```python
from build123d import *

# Parameters (mm, degrees)
ENL_V_MAT_EXTRU_1_DEPTH = 8.5
ESQUISSE3_R             = 1.25
ENL_V_MAT_EXTRU_2_DEPTH = 4
CHANFREIN1_SIZE         = 0.5


with BuildPart() as part:
    # Esquisse1 → Révolution1 (revolve)
    with BuildSketch(Plane.XY, mode=Mode.PRIVATE) as r_volution1_sk:
        Polygon((4.25, 1), (13.5, 1), (13.5, 22), (13.6, 22), (13.6, 37), (4.5, 37), (4.5, 41.5), (2, 41.5), (2, 52.5), (0, 52.5), (0, 0), (4.25, 0), align=None)
    revolve(r_volution1_sk.sketch.rotate(Axis((0, 52.5, 0), (0, -1, 0)), 180), axis=Axis((0, 52.5, 0), (0, -1, 0)))

    # Esquisse2 → Enlèv. mat.-Extru.1 (cut)
    with BuildSketch(Plane(origin=(0, 52.5, 0), x_dir=(1, 0, 0), z_dir=(0, 1, 0))):
        with BuildLine():
            Line((-1.322875656, 1.5), (1.322875656, 1.5))
            ThreePointArc((1.322875656, 1.5), (0, 2), (-1.322875656, 1.5))
        make_face()
    extrude(amount=-ENL_V_MAT_EXTRU_1_DEPTH, mode=Mode.SUBTRACT)

    # Esquisse3 → Enlèv. mat.-Extru.2 (cut)
    with BuildSketch(Plane(origin=(0, 37, 0), x_dir=(1, 0, 0), z_dir=(0, 1, 0))):
        with Locations(Location((0, 10, 0), (0, 0, 180))):
            Circle(ESQUISSE3_R)
        with Locations((0, -10)):
            Circle(ESQUISSE3_R)
    extrude(amount=-ENL_V_MAT_EXTRU_2_DEPTH, mode=Mode.SUBTRACT)

    # Chanfrein1
    chanfrein1_edges = [part.edges().sort_by_distance(p)[0] for p in [
        (13.6, 37, 0),
    ]]
    chamfer(chanfrein1_edges, length=CHANFREIN1_SIZE)


solid = part.part
```
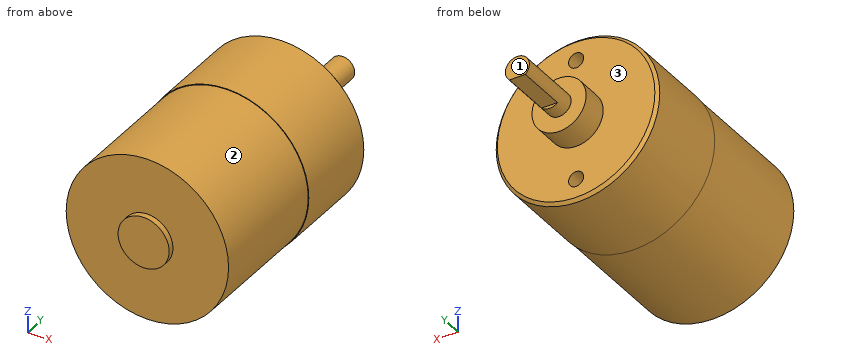
Geometry check sheet. Reference: the model listing, model coordinates, mm. Face numbers are marked on the shaded views. A direction names the side the tool comes from. Coordinates: 2 decimals unless noted, no trailing zeros. Write each loop counter-clockwise with the first axis right and the second up, starting at its lowest first coordinate (ties: lowest second). Pieces come first, ordered by that corner, then holes. Notation, with made-up numbers: M -18.5,5.5 L 10.5,5.5 A14 cw 10.5,18.5 Z; hole C 72,-6.75 d3. An arc over 180 degrees is marked long. Use one line per item in the form item = value. Start each with the question number.
1) Section check D-D on y = 46.5. Enter the section's corners in (x, z).
2) Section check C-C on y = 31.5. Enter the section's corners in (x, z).
3) Set-up check for the marked faces 1, 2 and 3: record each of +Z, -Z, +X, -X, +Y, -Y from which the full face is reachable in a straight line by a thin tool's end or side.
4) Go/stop test with flat-tipped pins: pin 1 Ø2 at (x, z) = (-2.5, -4.5) entering from +Y; pin 2 Ø10 at (y, z) = (16, -7.5) entering from +X; pin 3 Ø1.2 at (x, z) = (0.5, -9.5) entering from +Y. Record where each tip stops, or that it passes through.
5) Section check A-A on z = 0. Enter the section's corners in (x, y).
6) Thickness scan on probe 1 along Z at (x, y) = (0, 34.8); probe 2 along X at (y, z) = (21, -0.25); probe 3 along Y at (x, z) = (-4, 10.5). Record the ranges inside material, lowest first. Write a range as from..to.
Responses:
q1.outline = M -1.32,-1.5 L 1.32,-1.5 A2 ccw long Z
q2.outline = C 0,0 d27.2
q3.face_1 = +Z, -Z, +X, -X, +Y
q3.face_2 = -Y
q3.face_3 = +Y
q4.pin_1 = 41.5
q4.pin_2 = 13.27
q4.pin_3 = 37
q5.outline = M -13.6,22 L -13.5,22 L -13.5,1 L -4.25,1 L -4.25,0 L 4.25,0 L 4.25,1 L 13.5,1 L 13.5,22 L 13.6,22 L 13.6,36.5 L 13.1,37 L 4.5,37 L 4.5,41.5 L 2,41.5 L 2,52.5 L -2,52.5 L -2,41.5 L -4.5,41.5 L -4.5,37 L -13.1,37 L -13.6,36.5 Z
q6.probe_1 = -13.6..-11.25, -8.75..8.75, 11.25..13.6
q6.probe_2 = -13.5..13.5
q6.probe_3 = 1..37
